The listing builds one solid part. Answer for the finished solid, in the listing's coordinates (mm). A direction names the side the tool comes from. Give positions to 0.01 mm unless a question says otherwise; leave off trailing zeros. Write each loop counter-clockwise with the first axis right and the second up, starting at its lowest first coordinate (ties: lowest second). Pieces come first, ordered by that corner, then holes. Notation, with made-up numbers: M -26.5,71 L -2.5,71 A24 cw -2.5,84 Z; hole C 63.5,59.5 d2. An arc over 180 degrees is marked long. Return JSON: item names as keys, results as strings.
from build123d import *

# Parameters (mm, degrees)
F0_W     = 50.8
F0_H     = 50.8
F0_W_2   = 38.1
F0_H_2   = 38.1
F1_DEPTH = 254
F2_R     = 6.35
F3_R     = 6.35


with BuildPart() as f1:
    # F0 (on Top) → F1 (new body)
    with BuildSketch(Plane.XY):
        Rectangle(F0_W, F0_H)
        Rectangle(F0_W_2, F0_H_2, mode=Mode.SUBTRACT)
    extrude(amount=F1_DEPTH)

    # F2
    f2_edges = [f1.edges().sort_by_distance(p)[0] for p in [
        (-25.4, 25.4, 127),
        (-25.4, -25.4, 127),
        (19.05, -19.05, 127),
        (25.4, 25.4, 127),
        (-19.05, -19.05, 127),
        (-19.05, 19.05, 127),
        (19.05, 19.05, 127),
    ]]
    fillet(f2_edges, radius=F2_R)

    # F3
    f3_edges = [f1.edges().sort_by_distance(p)[0] for p in [
        (25.4, -25.4, 127),
    ]]
    fillet(f3_edges, radius=F3_R)


solid = f1.part
Item 1: Given pin 1 Ø2 at (x, y) = (12.5, 16.5) entering from +Z, flat-ended and moving along its own axis, determine where the tip first touches the part or whether it passes through.
Geometry results:
{"pin 1": "passes through"}
Item 2: A cutting plane is placed at A-A, the plane x = -9. Write down the section's boundary in (y, z), plus the area to 3 significant figures.
Geometry results:
{"outline": "M -25.4,0 L -19.05,0 L -19.05,254 L -25.4,254 Z; M 19.05,0 L 25.4,0 L 25.4,254 L 19.05,254 Z", "area": "3,230 mm2"}
Item 3: Which of the six approach directions +Z, -Z, +X, -X, +Y, -Y give full straight-line access (tool end or side, diameter ignored) to faces 4 (the cylindrical face through (17.24, 17.14, 128.78)), 5 (the flat face through (25.4, 0, 125))?
Geometry results:
{"face 4": "+Z, -Z", "face 5": "+Z, -Z, +X, +Y, -Y"}
Item 4: Find the intervals of material crossed by line 1 (X direction, y = 1, z = 60.5); line 2 (Y direction, x = -14, z = 132), in increasing order.
Geometry results:
{"line 1": "x = -25.4 to -19.05, 19.05 to 25.4", "line 2": "y = -25.4 to -18.92, 18.92 to 25.4"}
Item 5: Determine the mould class of faces 1 (the flat face through (0, 23, 254)), 2 (the cylindrical face through (-17.14, -17.24, 128.78)), 3 (the cylindrical face through (23.49, 23.59, 128.78)) for opening direction Y: +Y half, -Y half, draft (parallel to the pull), parting line (faces both ways), or undercut.
Geometry results:
{"face 1": "draft", "face 2": "undercut", "face 3": "+Y half"}
Item 6: A cutting plane is placed at D-D, the plane y = -21.5. Write down the section's boundary in (x, z), plus the area to 3 significant figures.
Geometry results:
{"outline": "M -24.91,0 L 24.91,0 L 24.91,254 L -24.91,254 Z", "area": "12,700 mm2"}
Item 7: A cutting plane is placed at C-C, the plane z = 190.5. Write down the section's boundary in (x, y).
Geometry results:
{"outline": "M -25.4,-19.05 A6.35 ccw -19.05,-25.4 L 19.05,-25.4 A6.35 ccw 25.4,-19.05 L 25.4,19.05 A6.35 ccw 19.05,25.4 L -19.05,25.4 A6.35 ccw -25.4,19.05 Z; hole M -19.05,-12.7 A6.35 ccw -12.7,-19.05 L 12.7,-19.05 A6.35 ccw 19.05,-12.7 L 19.05,12.7 A6.35 ccw 12.7,19.05 L -12.7,19.05 A6.35 ccw -19.05,12.7 Z"}
